Here's how the part is built. I have some questions about the finished solid (model axes, mm). A direction names the side the tool comes from. Coordinates: 2 decimals unless noted, no trailing zeros. Write each loop counter-clockwise with the first axis right and the second up, starting at its lowest first coordinate (ties: lowest second). Pieces come first, ordered by that corner, then holes. Notation, with made-up numbers: (-22.75, 28) - (-3.75, 28) arc R21 cw to (-3.75, 37) - close; hole circle Ø6 at (-17, 49). An arc over 180 degrees is marked (long way). Answer in a Markdown table with one row per item. Add a question column.
Item 1: We'd pull the mould along Y, two halves only. Please class faces 4 (the face through (14.99, 61.983, 3.168)), 5 (the face through (13.776, 11.352, 3.168)), 6 (the face through (0, 35, 15)), 7 (the face through (0, 0, 8)): +Y half, -Y half, draft (parallel to the pull), parting line (faces both ways), or undercut.
Item 2: Imagine slicing it at B-B (z = 0). Please give me the cut outline in (x, y), plus the area to 3 significant figures.
Item 3: Imagine slicing it at C-C (y = 10). Please give me the cut outline in (x, z).
Item 4: Imagine slicing it at D-D (x = -15.5). Please give me the cut outline in (y, z).
Item 5: Imagine slicing it at A-A (x = 0). Please give me the cut outline in (y, z).
Item 6: If I drill on probe 1 along Y at (x, z) = (15.25, 1.5); probe 2 along Z at (x, y) = (0, 59); probe 3 along Y at (x, z) = (-14, 5), over which ranges is the centre line in solid material (lowest first)? Write a range as from..to.
Item 7: I'm going to push flat-ended pins straight in: pin 1 (3 mm diameter, centred on x = -5.5, z = -8, fed in from -Y); pin 2 (2 mm diameter, centred on x = 1.5, y = 13.5, fed in from -Z); pin 3 (7.5 mm diameter, centred on x = 16.5, y = 52, fed in from -Z); pin 4 (8 mm diameter, centred on x = -10, y = 21, fed in from -Z). Where does each tip first touch, or does it pass through?
Item 8: Which directions (+Z, -Z, +X, -X, +Y, -Y) give clear straight access to the entire face, cutting with the end or side of a thin tool? Please do faces 1 (the face through (-14, 35, -9)), 2 (the face through (-21, 35, 3)), 3 (the face through (14, 35, -9)).
from build123d import *

# Parameters (mm, degrees)
F0_R     = 6
F1_DEPTH = 70
F2_R     = 2
F3_DEPTH = 26.001


with BuildPart() as f1:
    # F0 (on Front) → F1 (new body)
    with BuildSketch(Plane.XZ):
        with BuildLine():
            Line((21, 15), (-21, 15))
            Line((-21, 15), (-21, -9))
            Line((-21, -9), (-6.324555, -9))
            ThreePointArc((-6.324555, -9), (0, -11), (6.324555, -9))
            Line((6.324555, -9), (21, -9))
            Line((21, -9), (21, 15))
        make_face()
        Circle(F0_R, mode=Mode.SUBTRACT)
    extrude(amount=-F1_DEPTH)

    # F2 (on face) → F3 (cut, through all)
    with BuildSketch(Plane.XY.offset(15)):
        with Locations((-15.25, 10)):
            Circle(F2_R)
        with Locations((-15.25, 60)):
            Circle(F2_R)
        with Locations((15.25, 60)):
            Circle(F2_R)
        with Locations((15.25, 10)):
            Circle(F2_R)
    extrude(amount=-F3_DEPTH, mode=Mode.SUBTRACT)


solid = f1.part
Here are the results:
| question | item | result |
|---|---|---|
| 1 | face 4 | undercut |
| 1 | face 5 | undercut |
| 1 | face 6 | draft |
| 1 | face 7 | -Y half |
| 2 | outline | (-21, 0) - (-6, 0) - (-6, 70) - (-21, 70) - close; (6, 0) - (21, 0) - (21, 70) - (6, 70) - close; hole circle Ø4 at (-15.25, 10); hole circle Ø4 at (-15.25, 60); hole circle Ø4 at (15.25, 10); hole circle Ø4 at (15.25, 60) |
| 2 | area | 2,050 mm2 |
| 3 | outline | (-21, -9) - (-17.25, -9) - (-17.25, 15) - (-21, 15) - close; (-13.25, -9) - (-6.32, -9) arc R11 ccw to (6.32, -9) - (13.25, -9) - (13.25, 15) - (-13.25, 15) - close; (17.25, -9) - (21, -9) - (21, 15) - (17.25, 15) - close; hole circle Ø12 at (0, 0) |
| 4 | outline | (0, -9) - (8.02, -9) - (8.02, 15) - (0, 15) - close; (11.98, -9) - (58.02, -9) - (58.02, 15) - (11.98, 15) - close; (61.98, -9) - (70, -9) - (70, 15) - (61.98, 15) - close |
| 5 | outline | (0, -11) - (70, -11) - (70, -6) - (0, -6) - close; (0, 6) - (70, 6) - (70, 15) - (0, 15) - close |
| 6 | probe 1 | y = 0..8, 12..58, 62..70 |
| 6 | probe 2 | z = -11..-6, 6..15 |
| 6 | probe 3 | y = 0..8.44, 11.56..58.44, 61.56..70 |
| 7 | pin 1 | stops at y = 0 |
| 7 | pin 2 | stops at z = -10.99 |
| 7 | pin 3 | stops at z = -9 |
| 7 | pin 4 | stops at z = -9.22 |
| 8 | face 1 | -Z, -X, +Y, -Y |
| 8 | face 2 | +Z, -Z, -X, +Y, -Y |
| 8 | face 3 | -Z, +X, +Y, -Y |
